Verification items for the finished model (mm, model axes). Face numbers are marked on the shaded views. A direction names the side the tool comes from. Round coordinates to 2 decimals unless told otherwise and drop trailing zeros. Write each loop counter-clockwise with the first axis right and the second up, starting at its lowest first coordinate (ties: lowest second). Pieces come first, ordered by that corner, then holes. Notation, with made-up numbers: (14, 63.5) - (49, 63.5) arc R24 ccw to (49, 80.5) - close; hole circle Ø5 at (-12, 77.25). An arc over 180 degrees is marked (long way). Answer as a JSON object with one key per item and string values. Group by question number.
1) Section check A-A (y = -2.5). Enter the section's corners in (x, z), then the cut area to 3 significant figures.
2) Set-up check for the marked faces 1, 2 and 3: record each of +Z, -Z, +X, -X, +Y, -Y from which the full face is reachable in a straight line by a thin tool's end or side.
3) Go/stop test with flat-tipped pins: pin 1 Ø2 at (x, z) = (-1.5, -1.5) entering from -Y; pin 2 Ø4 at (x, y) = (0.5, 1) entering from +Z; pin 3 Ø1.5 at (x, z) = (-2, 0) entering from +Y. Record where each tip stops, or that it passes through.
4) Thickness scan on line 1 (Z direction, x = 0, y = 2.5); line 2 (Y direction, x = -1.5, z = 1.55); line 3 (Y direction, x = -1.75, z = 0.15). Record the ranges inside material, lowest first.
```python
from build123d import *

# Parameters (mm, degrees)
F0_R     = 0.75
F1_DEPTH = 3.35
F2_R     = 0.75
F3_DEPTH = 3.35


with BuildPart() as f1:
    # F0 (on Front) → F1 (new body, symmetric)
    with BuildSketch(Plane.XZ):
        Circle(F0_R)
    extrude(amount=F1_DEPTH, both=True)

    # F2 (on Right) → F3 (join, symmetric)
    with BuildSketch(Plane.YZ):
        Circle(F2_R)
    extrude(amount=F3_DEPTH, both=True)

    # F4 (on Top) → F5 (revolve)
    with BuildSketch(Plane.XY):
        with BuildLine():
            Line((0, 2.113225), (0, -2.336775))
            ThreePointArc((0, -2.336775), (2.354721, -0.111775), (0, 2.113225))
        make_face()
    revolve(axis=Axis((0, -0.111775, 0), (0, 1, 0)))


solid = f1.part
```
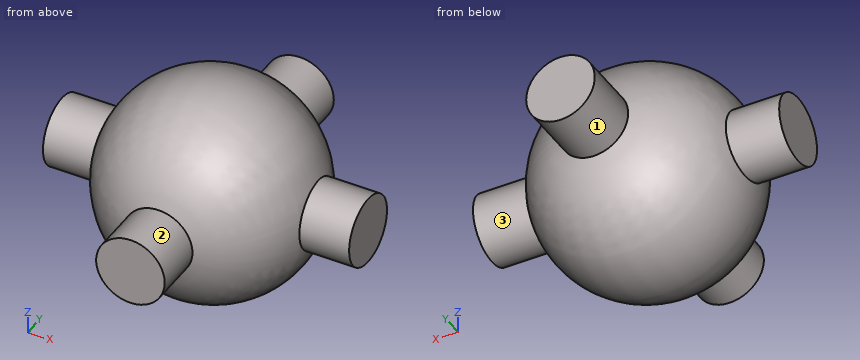
Returned:
{
 "1": {"outline": "circle Ø1.5 at (0, 0)", "area": "1.77 mm2"},
 "2": {"face 1": "+Y", "face 2": "-Y", "face 3": "+X"},
 "3": {"pin 1": "y = -2.11", "pin 2": "z = 2.35", "pin 3": "y = 1.81"},
 "4": {"line 1": "-0.75 to 0.75", "line 2": "-1.03 to 0.81", "line 3": "-1.63 to 1.41"}
}
